Can you work these out from the drawing? Everything is in mm from the part's minimum corner. Coordinates: 2 decimals unless noted, no trailing zeros. Answer as a JSON object with one key per item and string values.
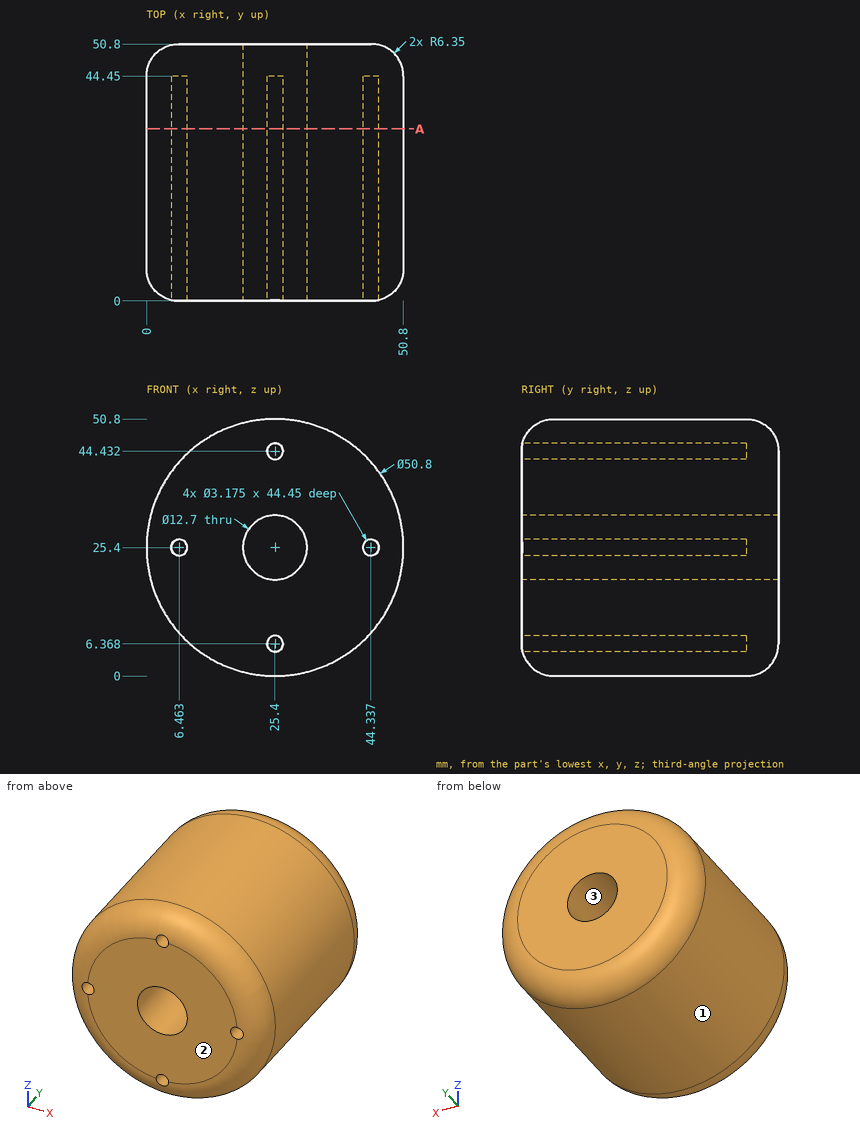
Item 1: If we mould it in two halves opening along X, with no side actions, what happens to the marked faces 1, 2 and 3? For each: pulls with the +X half, pulls with the -X half, needs draft (parallel to the pull), parting line crosses it, or undercut.
Answers follow:
{"face 1": "parting line crosses it", "face 2": "needs draft", "face 3": "undercut"}
Item 2: I'm going to push flat-ended pins straight in: pin 1 (2.5 mm diameter, centred on x = 24.5, z = 5.5, fed in from -Y); pin 2 (2.5 mm diameter, centred on x = 25.5, z = 44.5, fed in from -Y); pin 3 (7.5 mm diameter, centred on x = 25.4, z = 25.4, fed in from +Y); pin 4 (5 mm diameter, centred on y = 19.5, z = 9.5, fed in from -X). Where does each tip first touch, or does it pass through?
Answers follow:
{"pin 1": "stops at y = 0", "pin 2": "stops at y = 44.45", "pin 3": "passes through", "pin 4": "stops at x = 3.82"}
Item 3: Please list where these lines run through material, in increasing order: line 1 (Z direction, x = 25, y = 25) (1 decimal); line 2 (X direction, y = 40, z = 25); line 3 (X direction, y = 23, z = 26).
Answers follow:
{"line 1": "z = 0 to 4.8, 7.9 to 19.1, 31.7 to 42.9, 46 to 50.8", "line 2": "x = 0 to 4.93, 8 to 19.06, 31.74 to 42.8, 45.87 to 50.8", "line 3": "x = 0.01 to 4.99, 7.93 to 19.08, 31.72 to 42.87, 45.81 to 50.79"}
Item 4: I want a section at A-A, the plane y = 34. Give the number of separate pieces and of enclosed holes in the cut face, plus the area to 3 significant figures.
Answers follow:
{"separate pieces": "1", "enclosed holes": "5", "area": "1,870 mm^2"}
